Here's how the part is built. I have some questions about the finished solid (model axes, mm). A direction names the side the tool comes from. Round coordinates to 2 decimals unless told otherwise and drop trailing zeros.
```python
from build123d import *

# Parameters (mm, degrees)
EXTRUDE_1_DEPTH               = 3
HOLE_WIZARD_M2_1_AT_2_COUNT   = 2
HOLE_WIZARD_M2_1_AT_2_PITCH   = 21
PATTERN_LINEAR_1_COUNT        = 3
PATTERN_LINEAR_1_PITCH        = 33
PATTERN_LINEAR_2_COUNT        = 3
PATTERN_LINEAR_2_PITCH        = 10.5
PATTERN_LINEAR_3_COUNT        = 2
PATTERN_LINEAR_3_PITCH        = 31.5
HOLE_WIZARD_M2_1_2_AT_2_COUNT = 2
HOLE_WIZARD_M2_1_2_AT_2_PITCH = 16.970562748
SKETCH_8_R                    = 17
CUT_EXTRUDE_1_DEPTH           = 1
SKETCH_9_R                    = 2.025
CUT_EXTRUDE_2_DEPTH           = 75.994999833
PATTERN_CIRCULAR_1_COUNT      = 2
PATTERN_CIRCULAR_1_ANGLE      = 90
FILLET_1_R                    = 4
CHAMFER_1_SIZE                = 1


with BuildPart() as part:
    # ｽｹｯﾁ1 → ﾎﾞｽ - 押し出し1 (new body)
    with BuildSketch(Plane(origin=(0, 0, 0), x_dir=(1, 0, 0), z_dir=(0, 1, 0))):
        with BuildLine():
            Line((-10.05, 0), (-39, 0))
            Line((-39, 0), (-47.5, 8.5))
            Line((-47.5, 8.5), (-47.5, 58))
            Line((-47.5, 58), (47.5, 58))
            Line((47.5, 58), (47.5, 8.5))
            Line((47.5, 8.5), (39, 0))
            Line((39, 0), (10.05, 0))
            ThreePointArc((10.05, 0), (0, 10.05), (-10.05, 0))
        make_face()
    extrude(amount=EXTRUDE_1_DEPTH)

    # ｽｹｯﾁ3 → Hole Wizard M2 _1 (revolve, cut)
    with BuildSketch(Plane(origin=(-43.5, 3, -54), x_dir=(0, 0, 1), z_dir=(1, 0, 0))):
        Polygon((0, 0), (0, 4.63090365), (1.05, 4), (1.05, 1), (2, 1), (2, 0), align=None)
    hole_wizard_m2_1 = revolve(axis=Axis((-43.5, 9.35, -54), (0, -1, 0)), mode=Mode.SUBTRACT)

    # Hole Wizard M2 _1 at 2: Hole Wizard M2 _1 ×2
    with Locations(*[(i * HOLE_WIZARD_M2_1_AT_2_PITCH, 0, 0) for i in range(1, HOLE_WIZARD_M2_1_AT_2_COUNT)]):
        add(hole_wizard_m2_1, mode=Mode.SUBTRACT)

    # 直線ﾊﾟﾀｰﾝ1: Hole Wizard M2 _1 ×3
    with Locations(*[(i * PATTERN_LINEAR_1_PITCH, 0, 0) for i in range(1, PATTERN_LINEAR_1_COUNT)]):
        add(hole_wizard_m2_1, mode=Mode.SUBTRACT)

    # 直線ﾊﾟﾀｰﾝ1 copy 1 sketch → 直線ﾊﾟﾀｰﾝ1 copy 1 (revolve, cut)
    with BuildSketch(Plane(origin=(10.5, 3, -54), x_dir=(0, 0, 1), z_dir=(1, 0, 0))):
        Polygon((0, 0), (0, 4.63090365), (1.05, 4), (1.05, 1), (2, 1), (2, 0), align=None)
    revolve(axis=Axis((10.5, 9.35, -54), (0, -1, 0)), mode=Mode.SUBTRACT)

    # 直線ﾊﾟﾀｰﾝ1 copy 2 sketch → 直線ﾊﾟﾀｰﾝ1 copy 2 (revolve, cut)
    with BuildSketch(Plane(origin=(43.5, 3, -54), x_dir=(0, 0, 1), z_dir=(1, 0, 0))):
        Polygon((0, 0), (0, 4.63090365), (1.05, 4), (1.05, 1), (2, 1), (2, 0), align=None)
    revolve(axis=Axis((43.5, 9.35, -54), (0, -1, 0)), mode=Mode.SUBTRACT)

    # 直線ﾊﾟﾀｰﾝ2: Hole Wizard M2 _1 ×3
    with Locations(*[(0, 0, i * PATTERN_LINEAR_2_PITCH) for i in range(1, PATTERN_LINEAR_2_COUNT)]):
        add(hole_wizard_m2_1, mode=Mode.SUBTRACT)

    # 直線ﾊﾟﾀｰﾝ2 copy 1 sketch → 直線ﾊﾟﾀｰﾝ2 copy 1 (revolve, cut)
    with BuildSketch(Plane(origin=(-22.5, 3, -43.5), x_dir=(0, 0, 1), z_dir=(1, 0, 0))):
        Polygon((0, 0), (0, 4.63090365), (1.05, 4), (1.05, 1), (2, 1), (2, 0), align=None)
    revolve(axis=Axis((-22.5, 9.35, -43.5), (0, -1, 0)), mode=Mode.SUBTRACT)

    # 直線ﾊﾟﾀｰﾝ2 copy 2 sketch → 直線ﾊﾟﾀｰﾝ2 copy 2 (revolve, cut)
    with BuildSketch(Plane(origin=(-22.5, 3, -33), x_dir=(0, 0, 1), z_dir=(1, 0, 0))):
        Polygon((0, 0), (0, 4.63090365), (1.05, 4), (1.05, 1), (2, 1), (2, 0), align=None)
    revolve(axis=Axis((-22.5, 9.35, -33), (0, -1, 0)), mode=Mode.SUBTRACT)

    # 直線ﾊﾟﾀｰﾝ2 copy 3 sketch → 直線ﾊﾟﾀｰﾝ2 copy 3 (revolve, cut)
    with BuildSketch(Plane(origin=(-10.5, 3, -43.5), x_dir=(0, 0, 1), z_dir=(1, 0, 0))):
        Polygon((0, 0), (0, 4.63090365), (1.05, 4), (1.05, 1), (2, 1), (2, 0), align=None)
    revolve(axis=Axis((-10.5, 9.35, -43.5), (0, -1, 0)), mode=Mode.SUBTRACT)

    # 直線ﾊﾟﾀｰﾝ2 copy 4 sketch → 直線ﾊﾟﾀｰﾝ2 copy 4 (revolve, cut)
    with BuildSketch(Plane(origin=(-10.5, 3, -33), x_dir=(0, 0, 1), z_dir=(1, 0, 0))):
        Polygon((0, 0), (0, 4.63090365), (1.05, 4), (1.05, 1), (2, 1), (2, 0), align=None)
    revolve(axis=Axis((-10.5, 9.35, -33), (0, -1, 0)), mode=Mode.SUBTRACT)

    # 直線ﾊﾟﾀｰﾝ2 copy 5 sketch → 直線ﾊﾟﾀｰﾝ2 copy 5 (revolve, cut)
    with BuildSketch(Plane(origin=(22.5, 3, -43.5), x_dir=(0, 0, 1), z_dir=(1, 0, 0))):
        Polygon((0, 0), (0, 4.63090365), (1.05, 4), (1.05, 1), (2, 1), (2, 0), align=None)
    revolve(axis=Axis((22.5, 9.35, -43.5), (0, -1, 0)), mode=Mode.SUBTRACT)

    # 直線ﾊﾟﾀｰﾝ2 copy 6 sketch → 直線ﾊﾟﾀｰﾝ2 copy 6 (revolve, cut)
    with BuildSketch(Plane(origin=(22.5, 3, -33), x_dir=(0, 0, 1), z_dir=(1, 0, 0))):
        Polygon((0, 0), (0, 4.63090365), (1.05, 4), (1.05, 1), (2, 1), (2, 0), align=None)
    revolve(axis=Axis((22.5, 9.35, -33), (0, -1, 0)), mode=Mode.SUBTRACT)

    # 直線ﾊﾟﾀｰﾝ2 copy 7 sketch → 直線ﾊﾟﾀｰﾝ2 copy 7 (revolve, cut)
    with BuildSketch(Plane(origin=(10.5, 3, -43.5), x_dir=(0, 0, 1), z_dir=(1, 0, 0))):
        Polygon((0, 0), (0, 4.63090365), (1.05, 4), (1.05, 1), (2, 1), (2, 0), align=None)
    revolve(axis=Axis((10.5, 9.35, -43.5), (0, -1, 0)), mode=Mode.SUBTRACT)

    # 直線ﾊﾟﾀｰﾝ2 copy 8 sketch → 直線ﾊﾟﾀｰﾝ2 copy 8 (revolve, cut)
    with BuildSketch(Plane(origin=(10.5, 3, -33), x_dir=(0, 0, 1), z_dir=(1, 0, 0))):
        Polygon((0, 0), (0, 4.63090365), (1.05, 4), (1.05, 1), (2, 1), (2, 0), align=None)
    revolve(axis=Axis((10.5, 9.35, -33), (0, -1, 0)), mode=Mode.SUBTRACT)

    # 直線ﾊﾟﾀｰﾝ2 copy 9 sketch → 直線ﾊﾟﾀｰﾝ2 copy 9 (revolve, cut)
    with BuildSketch(Plane(origin=(43.5, 3, -43.5), x_dir=(0, 0, 1), z_dir=(1, 0, 0))):
        Polygon((0, 0), (0, 4.63090365), (1.05, 4), (1.05, 1), (2, 1), (2, 0), align=None)
    revolve(axis=Axis((43.5, 9.35, -43.5), (0, -1, 0)), mode=Mode.SUBTRACT)

    # 直線ﾊﾟﾀｰﾝ2 copy 10 sketch → 直線ﾊﾟﾀｰﾝ2 copy 10 (revolve, cut)
    with BuildSketch(Plane(origin=(43.5, 3, -33), x_dir=(0, 0, 1), z_dir=(1, 0, 0))):
        Polygon((0, 0), (0, 4.63090365), (1.05, 4), (1.05, 1), (2, 1), (2, 0), align=None)
    revolve(axis=Axis((43.5, 9.35, -33), (0, -1, 0)), mode=Mode.SUBTRACT)

    # 直線ﾊﾟﾀｰﾝ3: Hole Wizard M2 _1 ×2
    with Locations(*[(0, 0, i * PATTERN_LINEAR_3_PITCH) for i in range(1, PATTERN_LINEAR_3_COUNT)]):
        add(hole_wizard_m2_1, mode=Mode.SUBTRACT)

    # 直線ﾊﾟﾀｰﾝ3 copy 1 sketch → 直線ﾊﾟﾀｰﾝ3 copy 1 (revolve, cut)
    with BuildSketch(Plane(origin=(-22.5, 3, -22.5), x_dir=(0, 0, 1), z_dir=(1, 0, 0))):
        Polygon((0, 0), (0, 4.63090365), (1.05, 4), (1.05, 1), (2, 1), (2, 0), align=None)
    revolve(axis=Axis((-22.5, 9.35, -22.5), (0, -1, 0)), mode=Mode.SUBTRACT)

    # ｽｹｯﾁ5 → Hole Wizard M2 _1 2 (revolve, cut)
    with BuildSketch(Plane(origin=(-10.5, 3, -22.5), x_dir=(0, 0, 1), z_dir=(1, 0, 0))):
        Polygon((0, 0), (0, 6.480688495), (0.8, 6), (0.8, 0), align=None)
    hole_wizard_m2_1_2 = revolve(axis=Axis((-10.5, 9.35, -22.5), (0, -1, 0)), mode=Mode.SUBTRACT)

    # Hole Wizard M2 _1 2 at 2: Hole Wizard M2 _1 2 ×2
    with Locations(*[Vector(-0.7071067811865469, 0, 0.7071067811865482) * (i * HOLE_WIZARD_M2_1_2_AT_2_PITCH) for i in range(1, HOLE_WIZARD_M2_1_2_AT_2_COUNT)]):
        add(hole_wizard_m2_1_2, mode=Mode.SUBTRACT)

    # ｽｹｯﾁ7 → M2 なべ頭ねじ用座ぐり穴2 (revolve, cut)
    with BuildSketch(Plane(origin=(-43.5, 3, -12), x_dir=(0, 0, 1), z_dir=(1, 0, 0))):
        Polygon((0, 0), (0, 6.63090365), (1.05, 6), (1.05, 1), (2, 1), (2, 0), align=None)
    hole_wizard_m2_2 = revolve(axis=Axis((-43.5, 9.35, -12), (0, -1, 0)), mode=Mode.SUBTRACT)

    # ﾐﾗｰ1: Hole Wizard M2 _1 2, M2 なべ頭ねじ用座ぐり穴2 across plane
    add(hole_wizard_m2_1_2.mirror(Plane(origin=(0, 0, 0), x_dir=(0, 0, 1), z_dir=(1, 0, 0))), mode=Mode.SUBTRACT)
    add(hole_wizard_m2_2.mirror(Plane(origin=(0, 0, 0), x_dir=(0, 0, 1), z_dir=(1, 0, 0))), mode=Mode.SUBTRACT)

    # ﾐﾗｰ1 copy 1 sketch → ﾐﾗｰ1 copy 1 (revolve, cut)
    with BuildSketch(Plane(origin=(43.5, 3, -22.5), x_dir=(0, 0, 1), z_dir=(-1, 0, 0))):
        Polygon((0, 0), (0, -4.63090365), (1.05, -4), (1.05, -1), (2, -1), (2, 0), align=None)
    revolve(axis=Axis((43.5, 9.35, -22.5), (0, 1, 0)), mode=Mode.SUBTRACT)

    # ﾐﾗｰ1 copy 2 sketch → ﾐﾗｰ1 copy 2 (revolve, cut)
    with BuildSketch(Plane(origin=(22.5, 3, -22.5), x_dir=(0, 0, 1), z_dir=(-1, 0, 0))):
        Polygon((0, 0), (0, -4.63090365), (1.05, -4), (1.05, -1), (2, -1), (2, 0), align=None)
    revolve(axis=Axis((22.5, 9.35, -22.5), (0, 1, 0)), mode=Mode.SUBTRACT)

    # ﾐﾗｰ1 copy 3 sketch → ﾐﾗｰ1 copy 3 (revolve, cut)
    with BuildSketch(Plane(origin=(43.5, 3, -54), x_dir=(0, 0, 1), z_dir=(-1, 0, 0))):
        Polygon((0, 0), (0, -4.63090365), (1.05, -4), (1.05, -1), (2, -1), (2, 0), align=None)
    revolve(axis=Axis((43.5, 9.35, -54), (0, 1, 0)), mode=Mode.SUBTRACT)

    # ﾐﾗｰ1 copy 4 sketch → ﾐﾗｰ1 copy 4 (revolve, cut)
    with BuildSketch(Plane(origin=(22.5, 3, -54), x_dir=(0, 0, 1), z_dir=(-1, 0, 0))):
        Polygon((0, 0), (0, -4.63090365), (1.05, -4), (1.05, -1), (2, -1), (2, 0), align=None)
    revolve(axis=Axis((22.5, 9.35, -54), (0, 1, 0)), mode=Mode.SUBTRACT)

    # ﾐﾗｰ1 copy 5 sketch → ﾐﾗｰ1 copy 5 (revolve, cut)
    with BuildSketch(Plane(origin=(22.5, 3, -10.5), x_dir=(0, 0, 1), z_dir=(-1, 0, 0))):
        Polygon((0, 0), (0, -6.480688495), (0.8, -6), (0.8, 0), align=None)
    revolve(axis=Axis((22.5, 9.35, -10.5), (0, 1, 0)), mode=Mode.SUBTRACT)

    # ｽｹｯﾁ8 → ｶｯﾄ - 押し出し1 (cut)
    with BuildSketch(Plane(origin=(0, 3, 0), x_dir=(1, 0, 0), z_dir=(0, 1, 0))):
        Circle(SKETCH_8_R)
    extrude(amount=-CUT_EXTRUDE_1_DEPTH, mode=Mode.SUBTRACT)

    # ｽｹｯﾁ9 → ｶｯﾄ - 押し出し2 (cut, through all)
    with BuildSketch(Plane(origin=(0, 2, 0), x_dir=(1, 0, 0), z_dir=(0, 1, 0))):
        with Locations(Location((-9.899494937, 9.899494937, 0), (0, 0, 270))):
            Circle(SKETCH_9_R)
    cut_extrude_2 = extrude(amount=-CUT_EXTRUDE_2_DEPTH, mode=Mode.SUBTRACT)

    # 円形ﾊﾟﾀｰﾝ1: ｶｯﾄ - 押し出し2 ×2 about axis
    pattern_circular_1_axis = Axis((0, 3, 0), (0, -1, 0))
    for i in range(1, PATTERN_CIRCULAR_1_COUNT):
        add(cut_extrude_2.rotate(pattern_circular_1_axis, i * PATTERN_CIRCULAR_1_ANGLE / (PATTERN_CIRCULAR_1_COUNT - 1)), mode=Mode.SUBTRACT)

    # ﾌｨﾚｯﾄ1
    fillet_1_edges = [part.edges().sort_by_distance(p)[0] for p in [
        (-47.5, 1.5, -8.5),
        (-47.5, 1.5, -58),
        (47.5, 1.5, -58),
        (47.5, 1.5, -8.5),
        (39, 1.5, 0),
        (-39, 1.5, 0),
    ]]
    fillet(fillet_1_edges, radius=FILLET_1_R)

    # 面取り1
    chamfer_1_edges = [part.edges().sort_by_distance(p)[0] for p in [
        (0, 3, -17),
        (27.171572875, 3, 0),
        (38.87387948, 3, -0.30448187),
        (43.25, 3, -4.25),
        (47.19551813, 3, -8.62612052),
        (47.5, 3, -32.078427125),
        (-27.171572875, 3, 0),
        (46.328427125, 3, -56.828427125),
        (-38.87387948, 3, -0.30448187),
        (0, 3, -58),
        (-43.25, 3, -4.25),
        (-46.328427125, 3, -56.828427125),
        (-47.19551813, 3, -8.62612052),
        (-47.5, 3, -32.078427125),
    ]]
    chamfer(chamfer_1_edges, length=CHAMFER_1_SIZE - 0.0001)  # a hair under: the kernel refuses the full size


solid = part.part
```
1. I'm going to push a flat-ended pin straight in: P1, Ø3.5, axis at x = -43.5, z = -12, coming from the +Y side. Where does the tip first touch, or does it pass through?
Evaluation:
P1: stops at y = 2
2. On a 3-axis mill with a long thin cutter (end or side, diameter ignored), from which of +Z, -Z, +X, -X, +Y, -Y can I reach the whole of each face in a straight line? I mean faces 1 (the cylindrical face through (-11.13, 1.01, -11.51)), 2 (the cylindrical face through (41.548, 2.507, -22.934)). Say none if no direction works.
Evaluation:
face 1: +Y, -Y
face 2: +Y
3. I need wall thicknesses on probe 1 along Z at (x, y) = (-10.5, 1.25); probe 2 along X at (y, z) = (1.55, -11.5); probe 3 along Y at (x, z) = (22, -55). Which ranges of each line are inside material? Lowest first, please.
Evaluation:
probe 1: z = -58 to -55.05, -52.95 to -44.55, -42.45 to -34.05, -31.95 to -23.3, -21.7 to -11.83, -7.97 to 0
probe 2: x = -47.5 to -44.42, -42.58 to -11.14, -8.66 to 8.66, 11.14 to 42.58, 44.42 to 47.5
probe 3: y = 0 to 2
4. If we section it at B-B, the plane z = -43.5: State how many separate pieces and enclosed holes the cut face has, and give its area (3 significant figures).
Evaluation:
separate pieces: 7
enclosed holes: 0
area: 235 mm2
5. If we mould it in two halves opening along Z, with no side actions, what happens to faces 3 (the flat face through (-42.858, 2.493, -4.555)), 4 (the cylindrical face through (-41.548, 2.507, -12.434))? For each: released by +Z, released by -Z, zero draft, split by the parting line, or undercut.
Evaluation:
face 3: released by +Z
face 4: undercut
